from build123d import *

# Parameters (mm, degrees)
SKETCH_2_R            = 1.5
EXTRUDE_1_DEPTH       = 4
EXTRUDE_2_DEPTH       = 6
FILLET_1_R            = 0.1
HOLE_WIZARD_M31_D     = 2.5
HOLE_WIZARD_M31_DEPTH = 5
HOLE_WIZARD_M31_TIP   = 0.751075774
CHAMFER_2_SIZE        = 0.2


with BuildPart() as part:
    # Эскиз2 → Бобышка-Вытянуть1 (new body)
    with BuildSketch(Plane(origin=(0, 0, 0), x_dir=(1, 0, 0), z_dir=(0, 1, 0))):
        Circle(SKETCH_2_R)
    extrude(amount=EXTRUDE_1_DEPTH)

    # Эскиз3 → Бобышка-Вытянуть2 (add)
    with BuildSketch(Plane(origin=(0, 4, 0), x_dir=(1, 0, 0), z_dir=(0, 1, 0))):
        Polygon((-2.4, 1.385640646), (-2.4, -1.385640646), (0, -2.771281292), (2.4, -1.385640646), (2.4, 1.385640646), (0, 2.771281292), align=None)
    extrude(amount=EXTRUDE_2_DEPTH)

    # Скругление1
    fillet_1_edges = [part.edges().sort_by_distance(p)[0] for p in [
        (-1.2, 4, -2.078460969),
        (-2.4, 4, 0),
        (-1.2, 4, 2.078460969),
        (1.2, 4, 2.078460969),
        (2.4, 4, 0),
        (1.2, 4, -2.078460969),
        (-1.2, 10, -2.078460969),
        (-2.4, 10, 0),
        (-1.2, 10, 2.078460969),
        (1.2, 10, 2.078460969),
        (2.4, 10, 0),
        (1.2, 10, -2.078460969),
    ]]
    fillet(fillet_1_edges, radius=FILLET_1_R)

    # Отверстие обработанное метчиком M31
    with Locations(Plane.ZX.offset(10)):
        with Locations((0, 0)):
            Hole(HOLE_WIZARD_M31_D / 2, depth=HOLE_WIZARD_M31_DEPTH)
            with Locations((0, 0, -(HOLE_WIZARD_M31_DEPTH + HOLE_WIZARD_M31_TIP / 2))):  # 118° drill point
                Cone(0, HOLE_WIZARD_M31_D / 2, HOLE_WIZARD_M31_TIP, mode=Mode.SUBTRACT)

    # Фаска2
    chamfer_2_edges = [part.edges().sort_by_distance(p)[0] for p in [
        (-1.5, 0, 0),
        (0, 10, 1.25),
    ]]
    chamfer(chamfer_2_edges, length=CHAMFER_2_SIZE)


solid = part.part
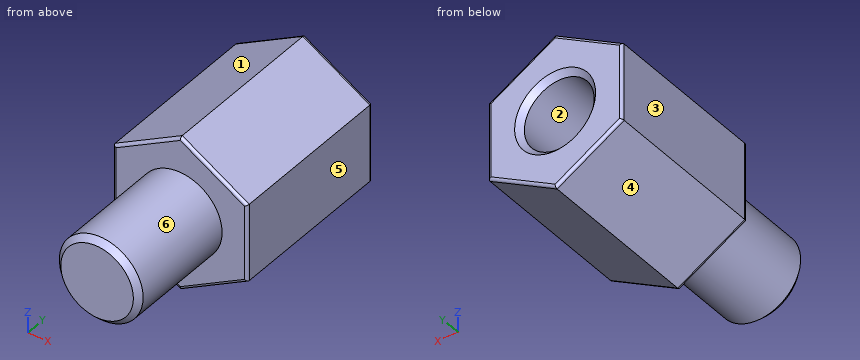
CAD build for the part. Positions are in the model's coordinates, mm. Face numbers are marked on the shaded views. A direction names the side the tool comes from. Round coordinates to 2 decimals unless told otherwise and drop trailing zeros. Loops run counter-clockwise (first coordinate to the right, second up) from the corner with the lowest first, then second, coordinate; pieces in that order, holes last. Notation, with made-up numbers: (9, -2) - (63, -2) arc R16 cw to (63, 17) - close; hole circle Ø1 at (-26.5, 17). An arc over 180 degrees is marked (long way). Put each result on its own line as item: value.
1. Wall check: line 1 (X direction, y = 7.45, z = 0); line 2 (Y direction, x = 1.35, z = 1.45); line 3 (Z direction, x = -1.05, y = 5.5). Give the ranges that are in metal, low to high.
Geometry check:
line 1: -2.4 to -1.25, 1.25 to 2.4
line 2: 4 to 10
line 3: -2.17 to -0.68, 0.68 to 2.17
2. Slice it at A-A on y = 6. List the corners of the cut face in (x, z), and give its area (3 significant figures).
Geometry check:
outline: (-2.4, -1.39) - (0, -2.77) - (2.4, -1.39) - (2.4, 1.39) - (0, 2.77) - (-2.4, 1.39) - close; hole circle Ø2.5 at (0, 0)
area: 15.0 mm²
3. Two-plate mould, pull along Z, no slides. Class the marked faces 1, 2, 3 and 4: released by +Z, released by -Z, zero draft, split by the parting line, or undercut.
Geometry check:
face 1: released by +Z
face 2: undercut
face 3: zero draft
face 4: released by -Z
4. 3-axis set-ups, long thin cutter, end or side, ignore diameter. For the marked faces 5 and 6: which of +Z, -Z, +X, -X, +Y, -Y reach the whole face in a straight line?
Geometry check:
face 5: +Z, -Z, +X, +Y, -Y
face 6: -Y
